```python
from build123d import *

# Parameters (mm, degrees)
F0_W     = 177.8
F0_H     = 47.6504
F1_DEPTH = 76.2
F2_R     = 4.7752
F2_R_2   = 1.9812
F3_DEPTH = 47.6514
F5_DEPTH = 16.002
F7_DEPTH = 33.528
F9_DEPTH = 31.7246


with BuildPart() as f1:
    # F0 (on Top) → F1 (new body)
    with BuildSketch(Plane.XY):
        with Locations((84.1375, 23.8252)):
            Rectangle(F0_W, F0_H)
    extrude(amount=-F1_DEPTH)

    # F2 (on Front) → F3 (cut, through all)
    with BuildSketch(Plane.XZ):
        with Locations((141.5288, -11.7856)):
            Circle(F2_R)
        with Locations((112.9538, -17.5006)):
            Circle(F2_R_2)
        with Locations((91.5416, -9.525)):
            Circle(F2_R_2)
    extrude(amount=-F3_DEPTH, mode=Mode.SUBTRACT)

    # F4 (on face) → F5 (cut)
    with BuildSketch(Plane.XY):
        with BuildLine():
            Line((172.1358, 22.1869), (172.1358, 25.4635))
            ThreePointArc((172.1358, 25.4635), (170.740896, 28.831096), (167.3733, 30.226))
            Line((167.3733, 30.226), (155.9433, 30.226))
            ThreePointArc((155.9433, 30.226), (152.575704, 28.831096), (151.1808, 25.4635))
            Line((151.1808, 25.4635), (151.1808, 22.1869))
            ThreePointArc((151.1808, 22.1869), (152.575704, 18.819304), (155.9433, 17.4244))
            Line((155.9433, 17.4244), (157.523438, 17.4244))
            Line((157.523438, 17.4244), (167.3733, 17.4244))
            ThreePointArc((167.3733, 17.4244), (170.740896, 18.819304), (172.1358, 22.1869))
        make_face()
    extrude(amount=-F5_DEPTH, mode=Mode.SUBTRACT)

    # F6 (on face) → F7 (cut)
    with BuildSketch(Plane.XY):
        with BuildLine():
            Line((113.0554, 27.781295), (103.7082, 27.781295))
            ThreePointArc((103.7082, 27.781295), (100.90636, 26.620735), (99.7458, 23.818895))
            ThreePointArc((99.7458, 23.818895), (100.90636, 21.017055), (103.7082, 19.856495))
            Line((103.7082, 19.856495), (113.0554, 19.856495))
            ThreePointArc((113.0554, 19.856495), (115.85724, 21.017055), (117.0178, 23.818895))
            ThreePointArc((117.0178, 23.818895), (115.85724, 26.620735), (113.0554, 27.781295))
        make_face()
    extrude(amount=-F7_DEPTH, mode=Mode.SUBTRACT)

    # F8 (on Top) → F9 (cut)
    with BuildSketch(Plane.XY):
        with BuildLine():
            Line((129.259735, 32.7152), (88.4682, 32.7152))
            ThreePointArc((88.4682, 32.7152), (84.552808, 31.093392), (82.931, 27.178))
            Line((82.931, 27.178), (82.931, 20.4724))
            ThreePointArc((82.931, 20.4724), (84.552808, 16.557008), (88.4682, 14.9352))
            Line((88.4682, 14.9352), (129.999633, 14.9352))
            ThreePointArc((129.999633, 14.9352), (132.65147, 15.611501), (134.655529, 17.4752))
            Line((134.655529, 17.4752), (134.611124, 28.6004))
            ThreePointArc((134.611124, 28.6004), (132.634974, 31.567573), (129.259735, 32.7152))
        make_face()
    extrude(amount=-F9_DEPTH, mode=Mode.SUBTRACT)


solid = f1.part
```
Input: part model. Units: mm. Frame: model coordinates. A direction names the side the tool comes from. Coordinates: 2 decimals unless noted, no trailing zeros. Loops run counter-clockwise (first coordinate to the right, second up) from the corner with the lowest first, then second, coordinate; pieces in that order, holes last. Notation, with made-up numbers: M 16,-35 L 60,-35 A22 cw 60,-8 Z; hole C 13.25,86 d8. An arc over 180 degrees is marked long. Use a Markdown table: item, result. Add a question column.
1) Section A-A, the plane z = -25. Return the cut outline in (x, y), plus the area to 3 significant figures.
2) Set-up query: faces 3 (the flat face through (-4.763, 23, -38)), 4 (the flat face through (108, 24, -33.528)). Return all of +Z, -Z, +X, -X, +Y, -Y with unobstructed straight access to the full face (end or side cutting, diameter ignored); none if empty.
3) Draft query along Y for faces 1 (the flat face through (83, 24, -76.2)), 2 (the cylindrical face through (84.51, 16.6, -15.64)). Return one class per face: +Y half, -Y half, draft (parallel to the pull), parting line (faces both ways), or undercut.
4) Line query: L1, parallel to Y at x = 123.5, z = -21; L2, parallel to X at y = 19, z = -6; L3, parallel to Z at x = 165.5, y = 19.5. Output: solid intervals per line, ascending. Write a range as from..to.
5) Section B-B, the plane x = 124. Return the cut outline in (y, z).
6) Pin query (flat end, axial travel): P1, Ø3, axis at x = 112.95, z = -17.5, coming from the +Y side. Return the tip coordinate at first contact, or that it passes through.
Answer below:
| question | item | result |
|---|---|---|
| 1 | outline | M -4.76,0 L 173.04,0 L 173.04,47.65 L -4.76,47.65 Z; hole M 82.93,20.47 A5.54 ccw 88.47,14.94 L 130,14.94 A5.54 ccw 134.66,17.48 L 134.61,28.6 A5.54 ccw 129.26,32.72 L 88.47,32.72 A5.54 ccw 82.93,27.18 Z |
| 1 | area | 7,580 mm2 |
| 2 | face 3 | +Z, -Z, -X, +Y, -Y |
| 2 | face 4 | +Z |
| 3 | face 1 | draft |
| 3 | face 2 | undercut |
| 4 | L1 | 0..14.94, 32.72..47.65 |
| 4 | L2 | -4.76..83.13, 134.65..152.4, 170.91..173.04 |
| 4 | L3 | -76.2..-16 |
| 5 | outline | M 0,-76.2 L 47.65,-76.2 L 47.65,0 L 32.72,0 L 32.72,-31.72 L 14.94,-31.72 L 14.94,0 L 0,0 Z |
| 6 | P1 | through |
